from build123d import *

# Parameters (mm, degrees)
SKETCH_W        = 38
SKETCH_H        = 36
PAD_DEPTH       = 2.5
SKETCH001_W     = 14
SKETCH001_H     = 14
POCKET_DEPTH    = 1.4
SKETCH002_W     = 15
SKETCH002_H     = 14
POCKET001_DEPTH = 1.1


with BuildPart() as part:
    # Sketch → Pad (new body)
    with BuildSketch(Plane.XY):
        Rectangle(SKETCH_W, SKETCH_H)
    extrude(amount=PAD_DEPTH)

    # Sketch001 (on DatumPlane) → Pocket (cut)
    with BuildSketch(Plane.XY.offset(2.5)):
        with Locations((-9, 8.5)):
            Rectangle(SKETCH001_W, SKETCH001_H)
        with Locations((9, 8.5)):
            Rectangle(SKETCH001_W, SKETCH001_H)
        with Locations((9, -8.5)):
            Rectangle(SKETCH001_W, SKETCH001_H)
        with Locations((-9, -8.5)):
            Rectangle(SKETCH001_W, SKETCH001_H)
    extrude(amount=-POCKET_DEPTH, mode=Mode.SUBTRACT)

    # Sketch002 → Pocket001 (cut)
    with BuildSketch(Plane.XY):
        with Locations((9, -8.5)):
            Rectangle(SKETCH002_W, SKETCH002_H)
        with Locations((9, 8.5)):
            Rectangle(SKETCH002_W, SKETCH002_H)
        with Locations((-9, 8.5)):
            Rectangle(SKETCH002_W, SKETCH002_H)
        with Locations((-9, -8.5)):
            Rectangle(SKETCH002_W, SKETCH002_H)
    extrude(amount=POCKET001_DEPTH, mode=Mode.SUBTRACT)


solid = part.part
Could you check a few things on this model? Use its own coordinates, in mm. A direction names the side the tool comes from. Give positions to 0.01 mm unless a question says otherwise; leave off trailing zeros. Order: outer loops, then holes, each group sorted by start corner. A loop starts at its lowest first (then second) coordinate and runs counter-clockwise, first axis right, second up.
1. Suppose I cut it at A-A (y = -11.5). List the corners of the cut face in (x, z) for me, plus the area to 3 significant figures.
2. We'd pull the mould along X, two halves only. Please class faces 1 (the flat face through (19, 0, 1)), 2 (the flat face through (9, 1.5, 1)), 3 (the flat face through (0, -18, 1)), 4 (the flat face through (-9, -1.5, 1)): pulls with the +X half, pulls with the -X half, needs draft (parallel to the pull), parting line crosses it, or undercut.
3. Will this pin go through, and if not, where does the flat tip stop? P1, Ø0.6, axis at x = 16, y = -11.5, coming from the -Z side.
4. Suppose I cut it at B-B (x = 12.5). List the corners of the cut face in (y, z) for me.
5. I need wall thicknesses on L1, parallel to X at y = 14.5, z = 1.9; L2, parallel to Y at x = 12.5, z = 1.4; L3, parallel to X at y = -14, z = 0.7. Which ranges of each line are inside material? Lowest first, please.
6. Suppose I cut it at C-C (z = 1.8). List the corners of the cut face in (x, y) for me, plus the area to 3 significant figures.
7. For faces 5 (the flat face through (16.5, 8.4, 0.5)), 6 (the flat face through (0, 0, 2.5)), 7 (the flat face through (-2, -9, 2)), which set-ups out of +Z, -Z, +X, -X, +Y, -Y let a thin tool reach every point of the face, with its end or its side?
Solved:
1. outline: (-19, 0) - (-16.5, 0) - (-16.5, 1.1) - (-16, 1.1) - (-16, 2.5) - (-19, 2.5) - close; (-2, 1.1) - (-1.5, 1.1) - (-1.5, 0) - (1.5, 0) - (1.5, 1.1) - (2, 1.1) - (2, 2.5) - (-2, 2.5) - close; (16, 1.1) - (16.5, 1.1) - (16.5, 0) - (19, 0) - (19, 2.5) - (16, 2.5) - close
1. area: 22.8 mm2
2. face 1: pulls with the +X half
2. face 2: undercut
2. face 3: needs draft
2. face 4: undercut
3. P1: stops at z = 1.1
4. outline: (-18, 0) - (-15.5, 0) - (-15.5, 2.5) - (-18, 2.5) - close; (-1.5, 0) - (1.5, 0) - (1.5, 2.5) - (-1.5, 2.5) - close; (15.5, 0) - (18, 0) - (18, 2.5) - (15.5, 2.5) - close
5. L1: x = -19 to -16, -2 to 2, 16 to 19
5. L2: y = -18 to -15.5, -1.5 to 1.5, 15.5 to 18
5. L3: x = -19 to -16.5, -1.5 to 1.5, 16.5 to 19
6. outline: (-19, -18) - (19, -18) - (19, 18) - (-19, 18) - close; hole (-16, -15.5) - (-2, -15.5) - (-2, -1.5) - (-16, -1.5) - close; hole (-16, 1.5) - (-2, 1.5) - (-2, 15.5) - (-16, 15.5) - close; hole (2, -15.5) - (16, -15.5) - (16, -1.5) - (2, -1.5) - close; hole (2, 1.5) - (16, 1.5) - (16, 15.5) - (2, 15.5) - close
6. area: 584 mm2
7. face 5: -Z
7. face 6: +Z, +X, -X, +Y, -Y
7. face 7: +Z, -Z
